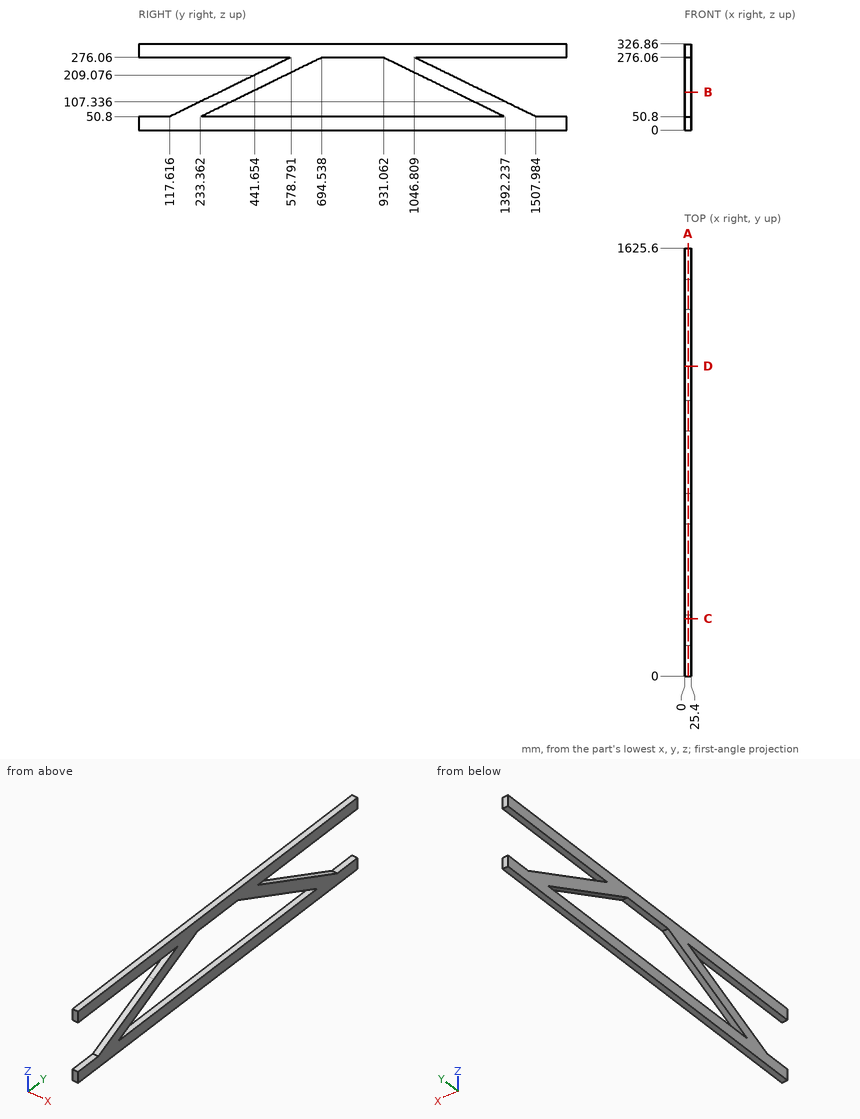
Check sheet for the drawn part. Datum: minimum x, y, z corner. Units: mm. Round coordinates to 2 decimals unless told otherwise and drop trailing zeros. Write each loop counter-clockwise with the first axis right and the second up, starting at its lowest first coordinate (ties: lowest second). Pieces come first, ordered by that corner, then holes. Notation, with made-up numbers: (-39.75, 71.5) -> (-13.75, 71.5) arc R16 ccw to (-13.75, 95.5) -> close; hole circle Ø4 at (80, 71.25). An arc over 180 degrees is marked (long way). One line per item, written item: value. Start each with the question number.
(1) Go/stop test with flat-tipped pins: pin 1 Ø12 at (x, z) = (10.5, 233) entering from +Y; pin 2 Ø5 at (x, z) = (13.5, 223.5) entering from +Y (1 decimal). Record where each tip stops, or that it passes through.
(2) Scan lines: line 1 (Z direction, x = 21.75, y = 1262.5) (1 decimal); line 2 (Z direction, x = 10.5, y = 291.5) (1 decimal); line 3 (Z direction, x = 14.5, y = 1543.5). Record each from-to range of solid material in increasing order. Write a range as [from, to].
(3) Cross-section at D-D, the plane y = 1177. Record the cut outline in (x, z).
(4) Cross-section at C-C, the plane y = 217.5. Record the cut outline in (x, z), and give its area (3 significant figures).
(5) Cross-section at B-B, the plane z = 144.5. Record the cut outline in (x, y) (1 decimal).
(6) Cross-section at A-A, the plane x = 13.5. Record the cut outline in (y, z) (1 decimal), and give its area (3 significant figures).
Answer:
1. pin 1: y = 1147.25
1. pin 2: y = 1159.5
2. line 1: [0, 50.8], [114.2, 170.7], [276.1, 326.9]
2. line 2: [0, 50.8], [79.2, 135.7], [276.1, 326.9]
2. line 3: [0, 50.8], [276.06, 326.86]
3. outline: (0, 0) -> (25.4, 0) -> (25.4, 50.8) -> (0, 50.8) -> close; (0, 155.93) -> (25.4, 155.93) -> (25.4, 212.47) -> (0, 212.47) -> close; (0, 276.06) -> (25.4, 276.06) -> (25.4, 326.86) -> (0, 326.86) -> close
4. outline: (0, 0) -> (25.4, 0) -> (25.4, 99.59) -> (0, 99.59) -> close; (0, 276.06) -> (25.4, 276.06) -> (25.4, 326.86) -> (0, 326.86) -> close
4. area: 3,820 mm²
5. outline: (0, 309.4) -> (25.4, 309.4) -> (25.4, 425.2) -> (0, 425.2) -> close; (0, 1200.4) -> (25.4, 1200.4) -> (25.4, 1316.2) -> (0, 1316.2) -> close
6. outline: (0, 0) -> (1625.6, 0) -> (1625.6, 50.8) -> (1508, 50.8) -> (1046.8, 276.1) -> (1625.6, 276.1) -> (1625.6, 326.9) -> (0, 326.9) -> (0, 276.1) -> (578.8, 276.1) -> (117.6, 50.8) -> (0, 50.8) -> close; hole (233.4, 50.8) -> (1392.2, 50.8) -> (931.1, 276.1) -> (694.5, 276.1) -> close
6. area: 217,000 mm²
